CAD build for the part. Positions are in the model's coordinates, mm. A direction names the side the tool comes from. Give positions to 0.01 mm unless a question says otherwise; leave off trailing zeros. Loops run counter-clockwise (first coordinate to the right, second up) from the corner with the lowest first, then second, coordinate; pieces in that order, holes last.
Item 1: Saw through at C-C on x = -5. Give the cut face in (y, z), plus the area to 3 significant figures.
Item 2: Mould opens along Y. For faces 1 (the flat face through (6.972, 54.346, 2.465)), 2 (the flat face through (0, 19, 0)), 3 (the cylindrical face through (4.284, 23.771, 2.465)) say: released by +Y, released by -Y, zero draft, split by the parting line, or undercut.
Item 3: Probe probe 1 along X at (y, z) = (30, 0.4); probe 2 along Y at (x, z) = (3.5, 2.8); probe 3 along Y at (x, z) = (2.75, 1.6). List the from-to ranges inside material, lowest first.
Item 4: Saw through at A-A on y = 0. Give the cut face in (x, z).
Item 5: Saw through at D-D on x = -2.5. Give the cut face in (y, z).
Item 6: Saw through at B-B on z = 2.45. Give the cut face in (x, y) (3 decimals), plus the area to 3 significant figures.
Item 7: Which spindle directions (+Z, -Z, +X, -X, +Y, -Y) get a long thin tool onto all of the face, cutting with end or side? Do faces 4 (the flat face through (-10, 0, 2)), 5 (the flat face through (8.022, 10.434, 2.465)). Say none if no direction does.
Item 8: Drop flat-ended pins along their axis: P1, Ø1, axis at y = 16.5, z = 3.5, coming from the -X side; P2, Ø2, axis at x = -5, y = 0, coming from the -Z side; P3, Ø1.5, axis at y = 35, z = 1, coming from the +X side; P4, Ø10, axis at x = 5.5, y = 33, coming from the +Z side. Give the stop position or say it passes through.
Autodesk Inventor part; units mm, degrees
ref_plane "YZ Plane" through (0, 0, 0) normal (1, 0, 0) x (0, 1, 0)
ref_plane "XZ Plane" through (0, 0, 0) normal (0, 1, 0) x (-1, 0, 0)
ref_plane "XY Plane" through (0, 0, 0) normal (0, 0, 1) x (1, 0, 0)
sketch "Sketch1" plane through (0, 0, 0) normal (0, 0, 1) x (1, 0, 0)
  line L0 (0, 0) -> (5, 0)
  line L1 (5, 0) -> (-5, 0)
  circle A0 centre (-5, 0) radius 1.75
  circle A1 centre (5, 0) radius 1.75
  line L2 (0, 0) -> (0, -5)
  line L3 (0, -5) -> (10, -5)
  line L4 (10, -5) -> (10, 5)
  line L5 (0, -5) -> (-10, -5)
  line L6 (-10, -5) -> (-10, 5)
  line L7 (10, 5) -> (5.9879, 16.023)
  line L8 (10, 5) -> (21.7305, 5) construction
  line L9 (4.7122, 31.9163) -> (8.5293, 51.8848)
  line L10 (7.5896, 53.9779) -> (6.3368, 54.7253)
  line L11 (-1.1361, 51.3703) -> (-10, 5)
  arc A2 (4.7122, 31.9163) -> (5.9879, 16.023) centre (34.1787, 26.2837) ccw
  arc A3 (8.5293, 51.8848) -> (7.5896, 53.9779) centre (6.5649, 52.2603) ccw
  arc A4 (6.3368, 54.7253) -> (-1.1361, 51.3703) centre (3.775, 50.4315) ccw
  point P0 (3.1596, 23.7939)
  point P1 (8.7922, 53.2603)
  point P2 (0.2046, 58.384)
  dimension "d0" = 5
  dimension "d1" = 10
  dimension "d2" = 3.5
  dimension "d3" = 3.5
  dimension "d4" = 5
  dimension "d5" = 10
  dimension "d6" = 10
  dimension "d7" = 10
  dimension "d8" = 10
  dimension "d9" = 20
  dimension "d10" = 110
  dimension "d11" = 30
  dimension "d12" = 10
  dimension "d13" = 110
  dimension "d14" = 30
  dimension "d15" = 2
  dimension "d16" = 5
extrude "Extrusion1" add sketch "Sketch1" along normal blind 5
properties part number "gripper"
Results below:
1. outline: (-5, 0) - (-1.75, 0) - (-1.75, 5) - (-5, 5) - close; (1.75, 0) - (31.16, 0) - (31.16, 5) - (1.75, 5) - close
1. area: 163 mm2
2. face 1: released by +Y
2. face 2: zero draft
2. face 3: undercut
3. probe 1: x = -5.22 to 4.41
3. probe 2: y = -5 to -0.9, 0.9 to 55.42
3. probe 3: y = -5 to 55.33
4. outline: (-10, 0) - (-6.75, 0) - (-6.75, 5) - (-10, 5) - close; (-3.25, 0) - (3.25, 0) - (3.25, 5) - (-3.25, 5) - close; (6.75, 0) - (10, 0) - (10, 5) - (6.75, 5) - close
5. outline: (-5, 0) - (44.24, 0) - (44.24, 5) - (-5, 5) - close
6. outline: (-10, -5) - (10, -5) - (10, 5) - (5.988, 16.023) arc R30.001 cw to (4.712, 31.916) - (8.529, 51.885) arc R2 ccw to (7.59, 53.978) - (6.337, 54.725) arc R5 ccw to (-1.136, 51.37) - (-10, 5) - close; hole circle Ø3.5 at (-5, 0); hole circle Ø3.5 at (5, 0)
6. area: 759 mm2
7. face 4: +Z, -Z, -X, +Y, -Y
7. face 5: +Z, -Z, +X
8. P1: stops at x = -7.9
8. P2: passes through
8. P3: stops at x = 5.45
8. P4: stops at z = 5
